Verification items for the finished model (mm, model axes). Face numbers are marked on the shaded views. A direction names the side the tool comes from. Round coordinates to 2 decimals unless told otherwise and drop trailing zeros. Write each loop counter-clockwise with the first axis right and the second up, starting at its lowest first coordinate (ties: lowest second). Pieces come first, ordered by that corner, then holes. Notation, with made-up numbers: (61, 55) - (116, 55) arc R8 cw to (116, 69) - close; hole circle Ø11 at (-38.75, -10.5). An arc over 180 degrees is marked (long way). Answer as a JSON object with one key per item and string values.
```python
from build123d import *

# Parameters (mm, degrees)
SKETCH1_W          = 68.58
SKETCH1_H          = 68.58
BASE_EXTRUDE_DEPTH = 104.14
SIDE_FILLETS_R     = 12.7
TOP_CUT_DEPTH      = 5.08
TOP_FACE_FILLET_R  = 1.27
SKETCH_TERMINALS_R = 6.35
TERMINALS_DEPTH    = 15.24
TERMINALS_TAPER    = 5


with BuildPart() as part:
    # Sketch1 → Base Extrude (new body)
    with BuildSketch(Plane(origin=(0, 0, 0), x_dir=(1, 0, 0), z_dir=(0, 1, 0))):
        Rectangle(SKETCH1_W, SKETCH1_H)
    extrude(amount=BASE_EXTRUDE_DEPTH)

    # Side Fillets
    side_fillets_edges = [part.edges().sort_by_distance(p)[0] for p in [
        (34.29, 52.07, 34.29),
        (-34.29, 52.07, 34.29),
        (-34.29, 52.07, -34.29),
        (34.29, 52.07, -34.29),
    ]]
    fillet(side_fillets_edges, radius=SIDE_FILLETS_R)

    # Sketch2 → Top Cut (cut)
    with BuildSketch(Plane(origin=(0, 104.14, 0), x_dir=(1, 0, 0), z_dir=(0, 1, 0))):
        with BuildLine():
            Line((-30.48, 21.59), (-30.48, -21.59))
            ThreePointArc((-30.48, -21.59), (-27.876179285, -27.876179285), (-21.59, -30.48))
            Line((-21.59, -30.48), (21.59, -30.48))
            ThreePointArc((21.59, -30.48), (27.876179285, -27.876179285), (30.48, -21.59))
            Line((30.48, -21.59), (30.48, 21.59))
            ThreePointArc((30.48, 21.59), (27.876179285, 27.876179285), (21.59, 30.48))
            Line((21.59, 30.48), (-21.59, 30.48))
            ThreePointArc((-21.59, 30.48), (-27.876179285, 27.876179285), (-30.48, 21.59))
        make_face()
    extrude(amount=-TOP_CUT_DEPTH, mode=Mode.SUBTRACT)

    # Top Face Fillet
    top_face_fillet_edges = [part.edges().sort_by_distance(p)[0] for p in [
        (0, 104.14, 34.29),
        (-34.29, 104.14, 0),
        (34.29, 104.14, 0),
        (0, 104.14, -34.29),
        (30.570256121, 104.14, 30.570256121),
        (30.570256121, 104.14, -30.570256121),
        (-30.570256121, 104.14, -30.570256121),
        (-30.570256121, 104.14, 30.570256121),
    ]]
    fillet(top_face_fillet_edges, radius=TOP_FACE_FILLET_R)

    # Sketch-TERMINALS → Terminals (add)
    with BuildSketch(Plane(origin=(0, 99.06, 0), x_dir=(1, 0, 0), z_dir=(0, 1, 0))):
        Circle(SKETCH_TERMINALS_R)
        with Locations((-17.960512242, 17.960512242)):
            Circle(SKETCH_TERMINALS_R)
    extrude(amount=TERMINALS_DEPTH, taper=TERMINALS_TAPER)


solid = part.part
```
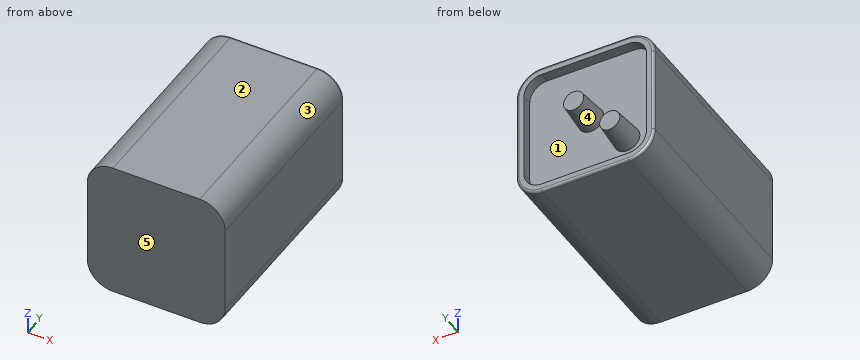
Q1. Section check B-B, the plane z = 10. Record the cut outline in (x, y), then the cut area to 3 significant figures.
Geometry check:
{"outline": "(-34.29, 0) - (34.29, 0) - (34.29, 102.87) arc R1.27 ccw to (33.02, 104.14) - (30.48, 104.14) - (30.48, 99.06) - (-30.48, 99.06) - (-30.48, 104.14) - (-33.02, 104.14) arc R1.27 ccw to (-34.29, 102.87) - close", "area": "6,830 mm2"}
Q2. Set-up check for the marked faces 1 and 2: record each of +Z, -Z, +X, -X, +Y, -Y from which the full face is reachable in a straight line by a thin tool's end or side.
Geometry check:
{"face 1": "+Y", "face 2": "+Z, +X, -X, +Y, -Y"}
Q3. Release check for a two-part mould opening along X. For the marked faces 3, 4 and 5 record: released by +X, released by -X, zero draft, split by the parting line, or undercut.
Geometry check:
{"face 3": "released by +X", "face 4": "undercut", "face 5": "zero draft"}
Q4. Section check C-C, the plane y = 97.5. Record the cut outline in (x, z).
Geometry check:
{"outline": "(-34.29, -21.59) arc R12.7 ccw to (-21.59, -34.29) - (21.59, -34.29) arc R12.7 ccw to (34.29, -21.59) - (34.29, 21.59) arc R12.7 ccw to (21.59, 34.29) - (-21.59, 34.29) arc R12.7 ccw to (-34.29, 21.59) - close"}
Q5. Section check D-D, the plane x = 15.5. Record the cut outline in (y, z).
Geometry check:
{"outline": "(0, -34.29) - (102.87, -34.29) arc R1.27 ccw to (104.14, -33.02) - (104.14, -30.48) - (99.06, -30.48) - (99.06, 30.48) - (104.14, 30.48) - (104.14, 33.02) arc R1.27 ccw to (102.87, 34.29) - (0, 34.29) - close"}
Q6. Section check A-A, the plane x = 0. Record the cut outline in (y, z), then the cut area to 3 significant figures.
Geometry check:
{"outline": "(0, -34.29) - (102.87, -34.29) arc R1.27 ccw to (104.14, -33.02) - (104.14, -30.48) - (99.06, -30.48) - (99.06, -6.35) - (114.3, -5.02) - (114.3, 5.02) - (99.06, 6.35) - (99.06, 30.48) - (104.14, 30.48) - (104.14, 33.02) arc R1.27 ccw to (102.87, 34.29) - (0, 34.29) - close", "area": "7,000 mm2"}
Q7. Material ranges on line 1 along Y through (x, z) = (22, -28); line 2 along Z through (x, y) = (-26, 76); line 3 along X through (y, z) = (77.5, -29.5), recorded low to high. Write a range as [from, to].
Geometry check:
{"line 1": "y = [0, 99.06]", "line 2": "z = [-33.5, 33.5]", "line 3": "x = [-31.53, 31.53]"}
